from build123d import *

# Parameters (mm, degrees)
F0_R     = 32.5
F0_R_2   = 1.5
F1_DEPTH = 26
F2_R     = 2.54
F4_DEPTH = 50.8
F5_R     = 1.27


with BuildPart() as f1:
    # F0 (on Front) → F1 (new body)
    with BuildSketch(Plane.XZ):
        Circle(F0_R)
        Circle(F0_R_2, mode=Mode.SUBTRACT)
    extrude(amount=F1_DEPTH)

    # F2
    f2_edges = [f1.edges().sort_by_distance(p)[0] for p in [
        (-32.5, -26, 0),
        (-32.5, 0, 0),
    ]]
    fillet(f2_edges, radius=F2_R)

    # F3 (on face) → F4 (cut)
    with BuildSketch(Plane.XZ.offset(26)):
        with BuildLine():
            Line((-1.512987, 6.16712), (-0.689091, 25.390651))
            ThreePointArc((-0.689091, 25.390651), (-7.849032, 24.156836), (-14.366764, 20.946505))
            Line((-14.366764, 20.946505), (-2.40091, 5.878617))
            ThreePointArc((-2.40091, 5.878617), (-1.962258, 6.039209), (-1.512987, 6.16712))
        make_face()
        with BuildLine():
            Line((2.40091, 5.878617), (14.366764, 20.946505))
            ThreePointArc((14.366764, 20.946505), (7.849032, 24.156836), (0.689091, 25.390651))
            Line((0.689091, 25.390651), (1.512987, 6.16712))
            ThreePointArc((1.512987, 6.16712), (1.962258, 6.039209), (2.40091, 5.878617))
        make_face()
        with BuildLine():
            Line((5.397741, 3.344681), (23.935003, 8.501507))
            ThreePointArc((23.935003, 8.501507), (20.549032, 14.929745), (15.481736, 20.136431))
            Line((15.481736, 20.136431), (4.848975, 4.099993))
            ThreePointArc((4.848975, 4.099993), (5.137258, 3.732436), (5.397741, 3.344681))
        make_face()
        with BuildLine():
            ThreePointArc((24.360885, -7.190779), (25.138879, -3.632735), (25.4, 0))
            ThreePointArc((25.4, 0), (25.138879, 3.632735), (24.360885, 7.190779))
            Line((24.360885, 7.190779), (6.332818, 0.466808))
            ThreePointArc((6.332818, 0.466808), (6.345703, 0.233562), (6.35, 0))
            ThreePointArc((6.35, 0), (6.345703, -0.233562), (6.332818, -0.466808))
            Line((6.332818, -0.466808), (24.360885, -7.190779))
        make_face()
        with BuildLine():
            ThreePointArc((15.481736, -20.136431), (20.549032, -14.929745), (23.935003, -8.501507))
            Line((23.935003, -8.501507), (5.397741, -3.344681))
            ThreePointArc((5.397741, -3.344681), (5.137258, -3.732436), (4.848975, -4.099993))
            Line((4.848975, -4.099993), (15.481736, -20.136431))
        make_face()
        with BuildLine():
            ThreePointArc((0.689091, -25.390651), (7.849032, -24.156836), (14.366764, -20.946505))
            Line((14.366764, -20.946505), (2.40091, -5.878617))
            ThreePointArc((2.40091, -5.878617), (1.962258, -6.039209), (1.512987, -6.16712))
            Line((1.512987, -6.16712), (0.689091, -25.390651))
        make_face()
        with BuildLine():
            ThreePointArc((-14.366764, -20.946505), (-7.849032, -24.156836), (-0.689091, -25.390651))
            Line((-0.689091, -25.390651), (-1.512987, -6.16712))
            ThreePointArc((-1.512987, -6.16712), (-1.962258, -6.039209), (-2.40091, -5.878617))
            Line((-2.40091, -5.878617), (-14.366764, -20.946505))
        make_face()
        with BuildLine():
            ThreePointArc((-23.935003, -8.501507), (-20.549032, -14.929745), (-15.481736, -20.136431))
            Line((-15.481736, -20.136431), (-4.848975, -4.099993))
            ThreePointArc((-4.848975, -4.099993), (-5.137258, -3.732436), (-5.397741, -3.344681))
            Line((-5.397741, -3.344681), (-23.935003, -8.501507))
        make_face()
        with BuildLine():
            Line((-6.332818, 0.466808), (-24.360885, 7.190779))
            ThreePointArc((-24.360885, 7.190779), (-25.4, 0), (-24.360885, -7.190779))
            Line((-24.360885, -7.190779), (-6.332818, -0.466808))
            ThreePointArc((-6.332818, -0.466808), (-6.35, 0), (-6.332818, 0.466808))
        make_face()
        with BuildLine():
            Line((-4.848975, 4.099993), (-15.481736, 20.136431))
            ThreePointArc((-15.481736, 20.136431), (-20.549032, 14.929745), (-23.935003, 8.501507))
            Line((-23.935003, 8.501507), (-5.397741, 3.344681))
            ThreePointArc((-5.397741, 3.344681), (-5.137258, 3.732436), (-4.848975, 4.099993))
        make_face()
    extrude(amount=-F4_DEPTH, mode=Mode.SUBTRACT)

    # F5
    f5_edges = [f1.edges().sort_by_distance(p)[0] for p in [
        (-1.5, -26, 0),
        (-1.5, 0, 0),
    ]]
    fillet(f5_edges, radius=F5_R)


solid = f1.part
Input: part model. Units: mm. Frame: model coordinates. Give positions to 0.01 mm unless a question says otherwise; leave off trailing zeros.
Q1. First-contact query: P1, Ø5, axis at y = -23, z = 25, coming from the +X side; P2, Ø5, axis at y = -22, z = -22, coming from the -X side; P3, Ø3.5, axis at x = 0, z = 0, coming from the +Y side. Flat tips, straight axial feed; report the tip coordinate or a pass-through.
Q2. Pull-direction query (Z, two-part tool) for faces 1 (the face through (14.54, -13.18, 5.89)), 2 (the face through (31, -12.85, 9.76)), 3 (the face through (0, 0, -6)); classes: pulls with the +Z half, pulls with the -Z half, needs draft (parallel to the pull), parting line crosses it, or undercut.
Q3. Material intervals for probe 1 along X at (y, z) = (-1.5, 20); probe 2 along Z at (x, y) = (21.5, -16.75); probe 3 along X at (y, z) = (-10.75, -22), sorted ascending.
Q4. Section A-A, the plane y = -21.25. State how many separate pieces and enclosed holes the cut face has, plus the area to 3 significant figures.
Filled in:
1. P1: stops at x = 23.45
1. P2: stops at x = -26
1. P3: stops at y = -0.51
2. face 1: undercut
2. face 2: parting line crosses it
2. face 3: needs draft
3. probe 1: x = -25.33 to -15.66, -15.39 to -13.62, -0.92 to 0.92, 13.62 to 15.39, 15.66 to 25.33
3. probe 2: z = -24.37 to -13.52, -7.82 to -6.12, 6.12 to 7.82, 13.52 to 24.37
3. probe 3: x = -23.92 to -12.69, -0.83 to 0.83, 12.69 to 23.92
4. separate pieces: 1
4. enclosed holes: 11
4. area: 1,830 mm2
